```python
from build123d import *

# Parameters (mm, degrees)
PAD_DEPTH         = 60
SKETCH001_R       = 3.1
POCKET_DEPTH      = 27.001
POCKET_DEPTH_BACK = -5.001
POCKET001_DEPTH   = 8.501
FILLET_R          = 2


with BuildPart() as part:
    # Sketch → Pad (new body)
    with BuildSketch(Plane.XZ):
        Polygon((-8.5, 5), (27, 5), (27, 0), (0, 0), (0, -27), (-8.5, -27), align=None)
    extrude(amount=PAD_DEPTH)

    # Sketch001 → Pocket (cut, two sides)
    with BuildSketch(Plane.XY) as pocket_sk:
        with Locations((14.811455, -51)):
            Circle(SKETCH001_R)
        with Locations((15, -9)):
            Circle(SKETCH001_R)
    extrude(amount=-POCKET_DEPTH, mode=Mode.SUBTRACT)
    extrude(pocket_sk.sketch, amount=-POCKET_DEPTH_BACK, mode=Mode.SUBTRACT)

    # Sketch002 → Pocket001 (cut, through all)
    with BuildSketch(Plane.YZ):
        with BuildLine():
            ThreePointArc((-52.5, -11.9), (-55.6, -15), (-52.5, -18.1))
            Line((-52.5, -18.1), (-49.5, -18.1))
            ThreePointArc((-49.5, -18.1), (-46.4, -15), (-49.5, -11.9))
            Line((-52.5, -11.9), (-49.5, -11.9))
        make_face()
        with BuildLine():
            ThreePointArc((-10.5, -11.9), (-13.6, -15), (-10.5, -18.1))
            Line((-10.5, -18.1), (-7.5, -18.1))
            ThreePointArc((-7.5, -18.1), (-4.4, -15), (-7.5, -11.9))
            Line((-10.5, -11.9), (-7.5, -11.9))
        make_face()
    extrude(amount=-POCKET001_DEPTH, mode=Mode.SUBTRACT)

    # Fillet
    fillet_edges = [part.edges().sort_by_distance(p)[0] for p in [
        (-4.25, -60, -27),
        (-4.25, 0, -27),
    ]]
    fillet(fillet_edges, radius=FILLET_R)


solid = part.part
```
The listing builds one solid part. Answer for the finished solid, in the listing's coordinates (mm). A direction names the side the tool comes from. Give positions to 0.01 mm unless a question says otherwise; leave off trailing zeros. Loops run counter-clockwise (first coordinate to the right, second up) from the corner with the lowest first, then second, coordinate; pieces in that order, holes last. Notation, with made-up numbers: M -28.75,23 L 26.25,23 A11 cw 26.25,39 Z; hole C 42.5,47 d7. An arc over 180 degrees is marked long. One line per item, written item: value.
1. Section C-C on x = 15 is taken. Determine the outline of the cut face in (y, z), plus the area to 3 significant figures.
Found:
outline: M -60,0 L -54.09,0 L -54.09,5 L -60,5 Z; M -47.91,0 L -12.1,0 L -12.1,5 L -47.91,5 Z; M -5.9,0 L 0,0 L 0,5 L -5.9,5 Z
area: 238 mm^2
2. For a pull along Z with two mould halves and no side action, classify faces 4 (the face through (-4, -9, -11.9)), 5 (the face through (-8.5, -30, -11)), 6 (the face through (-4.31, -59.43, -26.4)) as pulls with the +Z half, pulls with the -Z half, needs draft (parallel to the pull), parting line crosses it, or undercut.
Found:
face 4: undercut
face 5: needs draft
face 6: pulls with the -Z half
3. Find the intervals of material crossed by probe 1 along X at (y, z) = (-9, 2.2); probe 2 along Y at (x, z) = (15, 2.6); probe 3 along X at (y, z) = (-51, 2.45), in increasing order.
Found:
probe 1: -8.5 to 11.9, 18.1 to 27
probe 2: -60 to -54.09, -47.91 to -12.1, -5.9 to 0
probe 3: -8.5 to 11.71, 17.91 to 27
4. Section B-B on y = -9 is taken. Determine the outline of the cut face in (x, z).
Found:
outline: M -8.5,-27 L 0,-27 L 0,-18.1 L -8.5,-18.1 Z; M -8.5,-11.9 L 0,-11.9 L 0,0 L 11.9,0 L 11.9,5 L -8.5,5 Z; M 18.1,0 L 27,0 L 27,5 L 18.1,5 Z
5. For faces 1 (the face through (-4.2, -13.6, -14.9)), 2 (the face through (14, -30, 0)), 3 (the face through (-4.31, -0.57, -26.4)), determine the directions among +Z, -Z, +X, -X, +Y, -Y from which every point of the face is accessible in a straight line to the end or side of a thin tool.
Found:
face 1: +X, -X
face 2: -Z, +X, +Y, -Y
face 3: -Z, +X, -X, +Y
6. Each of these flat-tipped pins is pushed along its axis until it touches: P1, Ø12, axis at y = -31.5, z = -23.5, coming from the +X side; P2, Ø8, axis at x = 15, y = -9, coming from the -Z side. Where does it stop, or does it pass through?
Found:
P1: x = 0
P2: z = 0
7. Section A-A on x = -3 is taken. Determine the outline of the cut face in (y, z), plus the area to 3 significant figures.
Found:
outline: M -60,-25 A2 ccw -58,-27 L -2,-27 A2 ccw 0,-25 L 0,5 L -60,5 Z; hole M -52.5,-18.1 L -49.5,-18.1 A3.1 ccw -49.5,-11.9 L -52.5,-11.9 A3.1 ccw Z; hole M -10.5,-18.1 L -7.5,-18.1 A3.1 ccw -7.5,-11.9 L -10.5,-11.9 A3.1 ccw Z
area: 1,820 mm^2
8. Section D-D on z = 1.5 is taken. Determine the outline of the cut face in (x, y).
Found:
outline: M -8.5,-60 L 27,-60 L 27,0 L -8.5,0 Z; hole C 14.81,-51 d6.2; hole C 15,-9 d6.2
